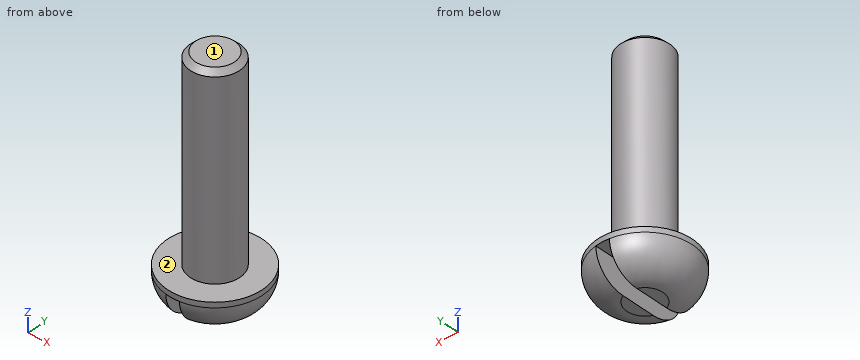
from build123d import *

# Parameters (mm, degrees)
ESBO_O1_R                = 4.5
RESSALTO_EXTRUS_O1_DEPTH = 3.3
ESBO_O2_R                = 2.35
RESSALTO_EXTRUS_O2_DEPTH = 22
FILETE1_R                = 2.8
ESBO_O3_W                = 1.3
ESBO_O3_H                = 10.03421546
CORTE_EXTRUS_O1_DEPTH    = 2.8
CHANFRO1_SIZE            = 0.5


with BuildPart() as part:
    # Esboço1 → Ressalto-extrusão1 (new body)
    with BuildSketch(Plane.XY):
        Circle(ESBO_O1_R)
    extrude(amount=RESSALTO_EXTRUS_O1_DEPTH)

    # Esboço2 → Ressalto-extrusão2 (add)
    with BuildSketch(Plane.XY):
        Circle(ESBO_O2_R)
    extrude(amount=RESSALTO_EXTRUS_O2_DEPTH)

    # Filete1
    filete1_edges = [part.edges().sort_by_distance(p)[0] for p in [
        (-4.5, 0, 0),
    ]]
    fillet(filete1_edges, radius=FILETE1_R)

    # Esboço3 → Corte-extrusão1 (cut)
    with BuildSketch(Plane(origin=(0, 0, 0), x_dir=(-1, 0, 0), z_dir=(0, 0, -1))):
        Rectangle(ESBO_O3_W, ESBO_O3_H)
    extrude(amount=-CORTE_EXTRUS_O1_DEPTH, mode=Mode.SUBTRACT)

    # Chanfro1
    chanfro1_edges = [part.edges().sort_by_distance(p)[0] for p in [
        (-2.35, 0, 22),
    ]]
    chamfer(chanfro1_edges, length=CHANFRO1_SIZE)


solid = part.part
The model under review builds one solid part; all positions refer to its coordinate system, in mm. Face numbers are marked on the shaded views. A direction names the side the tool comes from. Coordinates: 2 decimals unless noted, no trailing zeros. Write each loop counter-clockwise with the first axis right and the second up, starting at its lowest first coordinate (ties: lowest second). Pieces come first, ordered by that corner, then holes. Notation, with made-up numbers: (-29.5, 8) - (8.5, 8) arc R29 ccw to (8.5, 30) - close; hole circle Ø4 at (-38, 49). An arc over 180 degrees is marked (long way). Answer as a JSON object with one key per item and string values. Group by question number.
1. Add section A-A (x = 0). Give the boundary of the cut face in (y, z), plus the area to 3 significant figures.
2. Machinability: for the marked faces 1 and 2, which of the approach directions +Z, -Z, +X, -X, +Y, -Y give a long, thin tool a straight path to every point of the face, cutting with its end or side? Answer none if there is none.
3. Add section B-B (z = 10.75). Give the boundary of the cut face in (x, y).
4. Clearance check with flat-ended pins moving along their axes: pin 1 Ø1.5 at (y, z) = (2, 13) entering from -X; pin 2 Ø1.4 at (y, z) = (-2, 1.5) entering from -X; pin 3 Ø1.4 at (y, z) = (1, 1) entering from +X. State where each tip first meets the part, or that it passes through.
5. To check wall thickness, follow probe 1 along X at (y, z) = (-1.25, 1.5); probe 2 along X at (y, z) = (-2, 1.5); probe 3 along Z at (x, y) = (0.5, 3). State the ranges of each line that lie inside material, in increasing order.
Findings:
{
 "1": {"outline": "(-4.5, 2.8) - (4.5, 2.8) - (4.5, 3.3) - (2.35, 3.3) - (2.35, 21.5) - (1.85, 22) - (-1.85, 22) - (-2.35, 21.5) - (-2.35, 3.3) - (-4.5, 3.3) - close", "area": "92.1 mm²"},
 "2": {"face 1": "+Z, +X, -X, +Y, -Y", "face 2": "+Z"},
 "3": {"outline": "circle Ø4.7 at (0, 0)"},
 "4": {"pin 1": "x = -1.99", "pin 2": "x = -4.12", "pin 3": "x = 4.19"},
 "5": {"probe 1": "-3.99 to -0.65, 0.65 to 3.99", "probe 2": "-3.67 to -0.65, 0.65 to 3.67", "probe 3": "2.8 to 3.3"}
}
